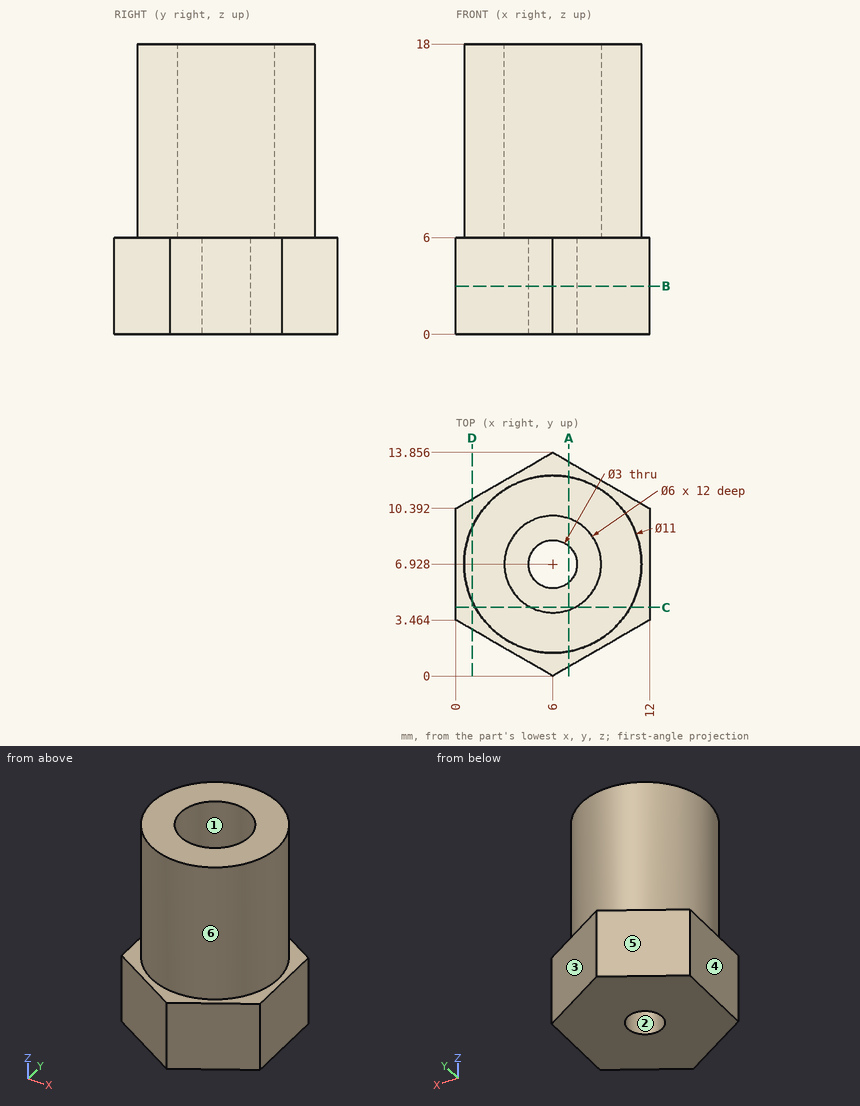
Job drawing, mm, ordinate dimensions from the low corner. One solid piece. A direction names the side the tool comes from. Coordinates: 2 decimals unless noted, no trailing zeros. Order: outer loops, then holes, each group sorted by start corner. A loop starts at its lowest first (then second) coordinate and runs counter-clockwise, first axis right, second up. Notation, with made-up numbers: (20.25, 28.25) - (62.25, 28.25) arc R20 cw to (62.25, 47.25) - close; hole circle Ø9 at (13, -35). An arc over 180 degrees is marked (long way). Write each question's results on one line, items separated by ' | '. Start each with the question number.
Item 1: Mould opens along X. For the marked faces 1, 2, 3 and 4 say: released by +X, released by -X, zero draft, split by the parting line, or undercut.
Item 2: Flat gauge pins, fed straight in: pin 1 (6.5 mm diameter, centred on x = 5.5, y = 8, fed in from +Z); pin 2 (1 mm diameter, centred on x = 5, z = 7, fed in from +Y) (1 decimal); pin 3 (4 mm diameter, centred on x = 9, z = 13.5, fed in from +Y); pin 4 (5 mm diameter, centred on x = 7.5, z = 13.5, fed in from -Y). Where does each tip first touch, or does it go through?
Item 3: Band-saw the part on B-B on z = 3. Write the cut outline in (x, y), and give its area (3 significant figures).
Item 4: Band-saw the part on A-A on x = 7. Write the cut outline in (y, z).
Item 5: Tool access for the marked faces 5 and 6: list every direction of +Z, -Z, +X, -X, +Y, -Y with a clear straight run to the whole face (end or side of a thin tool).
Item 6: Band-saw the part on D-D on x = 1. Write the cut outline in (y, z).
Item 7: Wall check: probe 1 along Y at (x, z) = (6, 12); probe 2 along X at (y, z) = (7.75, 13) (1 decimal); probe 3 along X at (y, z) = (6.75, 3.5). Give the ranges that are in metal, low to high. Write a range as [from, to].
Item 8: Band-saw the part on C-C on y = 4.25. Write the cut outline in (x, z).
Numbers:
1) face 1: undercut | face 2: undercut | face 3: released by +X | face 4: released by -X
2) pin 1: z = 18 | pin 2: y = 12.4 | pin 3: y = 12.34 | pin 4: y = 1.43
3) outline: (0, 3.46) - (6, 0) - (12, 3.46) - (12, 10.39) - (6, 13.86) - (0, 10.39) - close; hole circle Ø3 at (6, 6.93) | area: 118 mm^2
4) outline: (0.58, 0) - (5.81, 0) - (5.81, 6) - (4.1, 6) - (4.1, 18) - (1.52, 18) - (1.52, 6) - (0.58, 6) - close; (8.05, 0) - (13.28, 0) - (13.28, 6) - (12.34, 6) - (12.34, 18) - (9.76, 18) - (9.76, 6) - (8.05, 6) - close
5) face 5: +Z, -Z, -X, +Y | face 6: +Z
6) outline: (2.89, 0) - (10.97, 0) - (10.97, 6) - (9.22, 6) - (9.22, 18) - (4.64, 18) - (4.64, 6) - (2.89, 6) - close
7) probe 1: [1.43, 3.93], [9.93, 12.43] | probe 2: [0.6, 3.1], [8.9, 11.4] | probe 3: [0, 4.51], [7.49, 12]
8) outline: (0, 0) - (12, 0) - (12, 6) - (10.8, 6) - (10.8, 18) - (7.35, 18) - (7.35, 6) - (4.65, 6) - (4.65, 18) - (1.2, 18) - (1.2, 6) - (0, 6) - close
